```python
from build123d import *

# Parameters (mm, degrees)
F0_R          = 8.95
F1_DEPTH      = 0.75
F1_DEPTH_BACK = 0.75
F2_R          = 0.5
F4_R          = 2.75
F5_DEPTH      = 30.7
F5_DEPTH_BACK = 27


with BuildPart() as f1:
    # F0 (on Top) → F1 (new body, two sides)
    with BuildSketch(Plane.XY) as f1_sk:
        Circle(F0_R)
    extrude(amount=-F1_DEPTH)
    extrude(f1_sk.sketch, amount=F1_DEPTH_BACK)

    # F2 (on Front) → F3 (revolve, cut)
    with BuildSketch(Plane.XZ):
        with Locations((-8.8674183935, 0)):
            Circle(F2_R)
    revolve(axis=Axis((0, 0, -0.3013146343), (0, 0, -1)), mode=Mode.SUBTRACT)

    # F4 (on Top) → F5 (cut, two sides)
    with BuildSketch(Plane.XY) as f5_sk:
        Circle(F4_R)
    extrude(amount=-F5_DEPTH, mode=Mode.SUBTRACT)
    extrude(f5_sk.sketch, amount=F5_DEPTH_BACK, mode=Mode.SUBTRACT)


solid = f1.part
```
Here's how the part is built. I have some questions about the finished solid (model axes, mm). Coordinates: 2 decimals unless noted, no trailing zeros. Order: outer loops, then holes, each group sorted by start corner. A loop starts at its lowest first (then second) coordinate and runs counter-clockwise, first axis right, second up. Notation, with made-up numbers: (55, 79) - (86, 79) arc R32 cw to (86, 107) - close; hole circle Ø3 at (65.25, 27). An arc over 180 degrees is marked (long way). One line per question, with ' | ' between items. Start each with the question number.
1. Please list where these lines run through material, in increasing order: line 1 along Y through (x, z) = (0, 0.6); line 2 along X through (y, z) = (-2.5, 0.4); line 3 along Y through (x, z) = (0, 0.2). Write a range as [from, to].
2. If we section it at A-A (y = 0): Write out the boundary of the cut face in (x, z), and give its area (3 significant figures).
3. I'm going to push a flat-ended pin straight in: pin 1 Ø3.5 at (x, y) = (0, 0) entering from -Z. Where does the tip first touch, or does it pass through?
Model answer:
1) line 1: y = [-8.95, -2.75], [2.75, 8.95] | line 2: x = [-8.19, -1.15], [1.15, 8.19] | line 3: y = [-8.41, -2.75], [2.75, 8.41]
2) outline: (-8.95, -0.75) - (-2.75, -0.75) - (-2.75, 0.75) - (-8.95, 0.75) - (-8.95, 0.49) arc R0.5 cw (long way) to (-8.95, -0.49) - close; (2.75, -0.75) - (8.95, -0.75) - (8.95, -0.49) arc R0.5 cw (long way) to (8.95, 0.49) - (8.95, 0.75) - (2.75, 0.75) - close | area: 17.7 mm²
3) pin 1: passes through
